Model file for the job. Use its own axes, mm. A direction names the side the tool comes from. Coordinates: 2 decimals unless noted, no trailing zeros. Return JSON: item names as keys, results as strings.
Autodesk Inventor part; units mm, degrees
ref_plane "YZ Plane" through (0, 0, 0) normal (1, 0, 0) x (0, 1, 0)
ref_plane "XZ Plane" through (0, 0, 0) normal (0, 1, 0) x (-1, 0, 0)
ref_plane "XY Plane" through (0, 0, 0) normal (0, 0, 1) x (1, 0, 0)
sketch "BaseSC" plane through (0, 0, 0) normal (0, 1, 0) x (-1, 0, 0)
  line L0 (15, 13) -> (-15, 13)
  line L1 (-15, 13) -> (-15, -13)
  line L2 (-15, -13) -> (15, -13)
  line L3 (15, -13) -> (15, 13)
  line L4 (15, 13) -> (-15, -13) construction
  line L5 (-15, 13) -> (15, -13) construction
  line L6 (15, 13) -> (14.1667, 17.9301)
  line L7 (14.1667, 17.9301) -> (-15, 13)
  line L8 (0, 0) -> (8.3423, 0)
  line L9 (15, -13) -> (14.1667, -17.9301)
  line L10 (14.1667, -17.9301) -> (-15, -13)
  line L11 (-15, 13) -> (-14.1667, 17.9301)
  line L12 (-14.1667, 17.9301) -> (15, 13)
  dimension "d0" = 30
  dimension "d1" = 26
  dimension "d9" = 5
  dimension "d10" = 90
  dimension "d17" = 5
  dimension "d18" = 90
sketch "スケッチ2" plane through (0, 0, 0) normal (0, 0, 1) x (1, 0, 0)
  point P0 (0, 0)
extrude "押し出し1" add sketch "BaseSC" against normal blind 30 contours L3 L2 L1 L0
sketch "スケッチ3" plane through (15, 0, 13) normal (1, 0, 0) x (0, 0, -1)
  line L0 (2.5, -1.5742) -> (23.5, -1.5742)
  line L1 (23.5, -1.5742) -> (23.5, -28.5742)
  line L2 (23.5, -28.5742) -> (2.5, -28.5742)
  line L3 (2.5, -28.5742) -> (2.5, -1.5742)
  line L4 (2.5, -1.5742) -> (23.5, -28.5742) construction
  line L5 (23.5, -1.5742) -> (2.5, -28.5742) construction
  ellipse E0 centre (13, -15.0742) end of major axis (23.5, -15.0742) minor radius 13.5
  point P0 (13, 0)
  dimension "d5" = 21
  dimension "d6" = 27
extrude "押し出し2" cut sketch "スケッチ3" against normal through all contours E0
extrude "押し出し3" add sketch "BaseSC" along normal blind 36 contours L3 L2 L1 L0 | L9 L10 L2
extrude "押し出し5" add sketch "BaseSC" along normal blind 36 contours L0 L7 L12 | L11 L12 L7
sketch "スケッチ5" plane through (-14.1667, 0, -17.9301) normal (0.1666667, 0, -0.9860133) x (-0.9860133, 0, -0.1666667)
  circle A0 centre (-14.1422, 25) radius 5.3
  line L0 (-29.5804, 0) -> (0, 0)
  point P0 (-16.9569, 0)
  dimension "d21" = 10.6
  dimension "d22" = 25
extrude "押し出し6" cut sketch "スケッチ5" against normal through all
sketch "スケッチ6" plane through (0, -30, 0) normal (0, -1, 0) x (1, 0, 0)
  line L0 (15, -1) -> (-15, -1)
  line L1 (-15, -1) -> (-15, 1)
  line L2 (-15, 1) -> (15, 1)
  line L3 (15, 1) -> (15, -1)
  line L4 (15, -1) -> (-15, 1) construction
  line L5 (-15, -1) -> (15, 1) construction
  point P0 (0, 0)
  dimension "d25" = 30
  dimension "d26" = 2
extrude "押し出し7" cut sketch "スケッチ6" against normal blind 5
fillet "フィレット1" radius 10 2 edges at (15, 36, 0) (-15, 36, 0)
sketch "スケッチ7" plane through (-14.1667, 0, -17.9301) normal (0.1666667, 0, -0.9860133) x (-0.9860133, 0, -0.1666667)
  circle A0 centre (-14.1422, 25) radius 5.3
  ellipse E0 centre (-9.2967, 26) end of major axis (0.8452, 26) minor radius 10 (0, 29.9965) -> (-9.2967, 36) ccw
  line L0 (-19.4385, 36) -> (-9.2967, 36)
  ellipse E1 centre (-19.4385, 26) end of major axis (-29.5804, 26) minor radius 10 (-19.4385, 36) -> (-29.5804, 26) ccw
  line L1 (-29.5804, 0) -> (-29.5804, 26)
  line L2 (-29.5804, 0) -> (0, 0)
  line L3 (0, 0) -> (0, 29.9965)
  point P0 (-16.9569, 0)
extrude "押し出し8" cut sketch "スケッチ7" against normal through all
sketch "スケッチ8" plane through (14.1667, 0, 17.9301) normal (-0.1666667, 0, 0.9860133) x (0.9860133, 0, 0.1666667)
  line L0 (-4.3333, 26) -> (-4.3333, 0)
  line L1 (-4.3333, 0) -> (0, 0)
  line L2 (0, 0) -> (0, 29.9965)
  ellipse E0 centre (-9.2967, 26) end of major axis (0.8452, 26) minor radius 10 (0, 29.9965) -> (-9.2967, 36) ccw
  line L3 (-14.4752, 36) -> (-9.2967, 36)
  ellipse E1 centre (-14.4752, 26) end of major axis (-4.3333, 26) minor radius 10 (-4.3333, 26) -> (-14.4752, 36) ccw
  point P0 (-16.9569, 0)
extrude "押し出し9" cut sketch "スケッチ8" against normal through all
properties part number "default"
Item 1: 3-axis set-ups, long thin cutter, end or side, ignore diameter. For faces 1 (the flat face through (0, -15, 13)), 2 (the flat face through (0, -29, 1)): which of +Z, -Z, +X, -X, +Y, -Y reach the whole face in a straight line?
Check result:
{"face 1": "+Z, +X, -X, +Y, -Y", "face 2": "+X, -X, -Y"}
Item 2: Wall check: line 1 (Z direction, x = -9, y = -11.5); line 2 (Y direction, x = 9.5, z = -4.75); line 3 (Z direction, x = -5, y = -12). Give the ranges that are in metal, low to high.
Check result:
{"line 1": "z = -13 to -10.13, 10.13 to 13", "line 2": "y = -30 to -27.11, -3.03 to 0", "line 3": "z = -13 to -10.22, 10.22 to 13"}
Item 3: Pull direction Z, two halves, no side cores. Call faces 3 (the flat face through (0, -15, -13)), 4 (the flat face through (0, -30, -7)), 5 (the flat face through (0, -29, -1)): +Z half, -Z half, draft (parallel to the pull), parting line (faces both ways), or undercut.
Check result:
{"face 3": "-Z half", "face 4": "draft", "face 5": "undercut"}
